CAD build for the part. Positions are in the model's coordinates, mm. Face numbers are marked on the shaded views. A direction names the side the tool comes from. Coordinates: 2 decimals unless noted, no trailing zeros. Loops run counter-clockwise (first coordinate to the right, second up) from the corner with the lowest first, then second, coordinate; pieces in that order, holes last.
1) Pin check, flat tips, straight feed: pin 1 Ø1.5 at (x, y) = (-13, 1) entering from +Z; pin 2 Ø1.5 at (x, y) = (13, 1.5) entering from -Z; pin 3 Ø1 at (x, y) = (2.5, 2) entering from +Z; pin 4 Ø2 at (x, z) = (-2.5, -11.5) entering from -Y. Stop position of each tip, or through.
2) Saw through at C-C, the plane x = 9. Write the cut outline in (y, z).
3) Saw through at A-A, the plane y = 1.6. Write the cut outline in (x, z).
4) Saw through at B-B, the plane z = -9. Write the cut outline in (x, y), and give its area (3 significant figures).
5) Which spindle directions (+Z, -Z, +X, -X, +Y, -Y) get a long thin tool onto all of the face, cutting with end or side? Do the marked faces 1, 2 and 3. Say none if no direction does.
6) Wall check: line 1 along Z through (x, y) = (6.5, 2.1); line 2 along Z through (x, y) = (3.5, 2.4); line 3 along X through (y, z) = (1.25, -2.75). Give the ranges that are in metal, low to high.
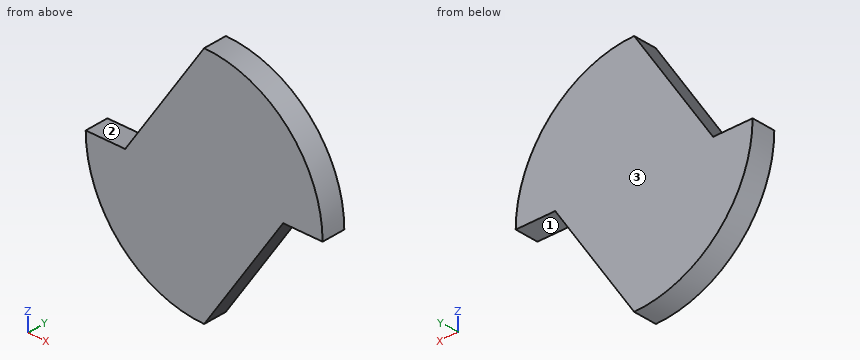
```python
from build123d import *

# Parameters (mm, degrees)
SKETCH1_R           = 15
BOSS_EXTRUDE1_DEPTH = 3
CUT_EXTRUDE2_START  = -8
CUT_EXTRUDE2_DEPTH  = 8


with BuildPart() as part:
    # Sketch1 → Boss-Extrude1 (new body)
    with BuildSketch(Plane(origin=(0, 0, 0), x_dir=(1, 0, 0), z_dir=(0, 1, 0))):
        with Locations(Location((0, 0, 0), (0, 0, 270))):
            Circle(SKETCH1_R)
    extrude(amount=BOSS_EXTRUDE1_DEPTH)

    # Sketch3 → Cut-Extrude2 (cut)
    with BuildSketch(Plane(origin=(0, 3, 0), x_dir=(1, 0, 0), z_dir=(0, 1, 0)).offset(CUT_EXTRUDE2_START)):
        with BuildLine():
            Line((0, -15), (-10, 0))
            Line((-10, 0), (-15, 0))
            ThreePointArc((-15, 0), (-10.606601718, -10.606601718), (0, -15))
        make_face()
        with BuildLine():
            Line((0, 15), (10, 0))
            Line((10, 0), (15, 0))
            ThreePointArc((15, 0), (10.606601718, 10.606601718), (0, 15))
        make_face()
    extrude(amount=CUT_EXTRUDE2_DEPTH, mode=Mode.SUBTRACT)


solid = part.part
```
Data:
1. pin 1: stops at z = 0
1. pin 2: stops at z = 0
1. pin 3: stops at z = 14.87
1. pin 4: stops at y = 0
2. outline: (0, -1.5) - (3, -1.5) - (3, 12) - (0, 12) - close
3. outline: (-15, 0) arc R15 ccw to (0, -15) - (10, 0) - (15, 0) arc R15 ccw to (0, 15) - (-10, 0) - close
4. outline: (-12, 0) - (4, 0) - (4, 3) - (-12, 3) - close
4. area: 48.0 mm2
5. face 1: -Z, +X, +Y, -Y
5. face 2: +Z, -X, +Y, -Y
5. face 3: +Z, -Z, +X, -X, +Y
6. line 1: z = -5.25 to 13.52
6. line 2: z = -9.75 to 14.59
6. line 3: x = -14.75 to 8.17
